```python
from build123d import *

# Parameters (mm, degrees)
SKETCH1_W                 = 82.55
SKETCH1_H                 = 12.7
BOSS_EXTRUDE1_DEPTH       = 3.175
SKETCH3_W                 = 12.7
SKETCH3_H                 = 12.7
BOSS_EXTRUDE2_DEPTH       = 38.1
SKETCH4_W                 = 12.7
SKETCH4_H                 = 12.7
BOSS_EXTRUDE3_DEPTH       = 38.1
SKETCH5_W                 = 6.858
SKETCH5_H                 = 6.858
CUT_EXTRUDE1_DEPTH        = 38.1
SKETCH6_W                 = 6.858
SKETCH6_H                 = 6.858
CUT_EXTRUDE2_DEPTH        = 38.1
SKETCH9_R                 = 2.54
CUT_EXTRUDE3_DEPTH        = 38.1
F_8_32_TAPPED_HOLE2_D     = 3.4544
F_8_32_TAPPED_HOLE2_DEPTH = 2.921


with BuildPart() as part:
    # Sketch1 → Boss-Extrude1 (new body)
    with BuildSketch(Plane(origin=(0, 0, 0), x_dir=(1, 0, 0), z_dir=(0, 1, 0))):
        Rectangle(SKETCH1_W, SKETCH1_H)
    extrude(amount=BOSS_EXTRUDE1_DEPTH)

    # Sketch3 → Boss-Extrude2 (add)
    with BuildSketch(Plane(origin=(0, 3.175, 0), x_dir=(1, 0, 0), z_dir=(0, 1, 0))):
        with Locations((-34.925, 0)):
            Rectangle(SKETCH3_W, SKETCH3_H)
    extrude(amount=BOSS_EXTRUDE2_DEPTH)

    # Sketch4 → Boss-Extrude3 (add)
    with BuildSketch(Plane(origin=(0, 3.175, 0), x_dir=(1, 0, 0), z_dir=(0, 1, 0))):
        with Locations((34.925, 0)):
            Rectangle(SKETCH4_W, SKETCH4_H)
    extrude(amount=BOSS_EXTRUDE3_DEPTH)

    # Sketch5 → Cut-Extrude1 (cut)
    with BuildSketch(Plane(origin=(0, 41.275, 0), x_dir=(1, 0, 0), z_dir=(0, 1, 0))):
        with Locations((-34.925, 0)):
            Rectangle(SKETCH5_W, SKETCH5_H)
    extrude(amount=-CUT_EXTRUDE1_DEPTH, mode=Mode.SUBTRACT)

    # Sketch6 → Cut-Extrude2 (cut)
    with BuildSketch(Plane(origin=(0, 41.275, 0), x_dir=(1, 0, 0), z_dir=(0, 1, 0))):
        with Locations((34.925, 0)):
            Rectangle(SKETCH6_W, SKETCH6_H)
    extrude(amount=-CUT_EXTRUDE2_DEPTH, mode=Mode.SUBTRACT)

    # Sketch9 → Cut-Extrude3 (cut)
    with BuildSketch(Plane(origin=(0, 3.175, 0), x_dir=(1, 0, 0), z_dir=(0, 1, 0))):
        with Locations(Location((-16.51, 0, 0), (0, 0, 270))):
            Circle(SKETCH9_R)
        with Locations(Location((16.51, 0, 0), (0, 0, 270))):
            Circle(SKETCH9_R)
    extrude(amount=-CUT_EXTRUDE3_DEPTH, mode=Mode.SUBTRACT)

    # #8-32 Tapped Hole2
    with Locations(Plane(origin=(-34.925, 36.83, 6.35), x_dir=(1, 0, 0), z_dir=(0, 0, 1))):
        with Locations((0, 0), (69.85, 0)):
            Hole(F_8_32_TAPPED_HOLE2_D / 2, depth=F_8_32_TAPPED_HOLE2_DEPTH)


solid = part.part
```
Here's how the part is built. I have some questions about the finished solid (model axes, mm). A direction names the side the tool comes from. Coordinates: 2 decimals unless noted, no trailing zeros. Loops run counter-clockwise (first coordinate to the right, second up) from the corner with the lowest first, then second, coordinate; pieces in that order, holes last. Notation, with made-up numbers: (16, 48.5) -> (40, 48.5) arc R31 ccw to (40, 76.5) -> close; hole circle Ø4 at (55.5, 78.25). An arc over 180 degrees is marked (long way). Return JSON: item names as keys, results as strings.
1) If we section it at A-A, the plane y = 6: Write out the boundary of the cut face in (x, z) (3 decimals).
Results below:
{"outline": "(-41.275, -6.35) -> (-28.575, -6.35) -> (-28.575, 6.35) -> (-41.275, 6.35) -> close; (28.575, -6.35) -> (41.275, -6.35) -> (41.275, 6.35) -> (28.575, 6.35) -> close; hole (-38.354, -3.429) -> (-31.496, -3.429) -> (-31.496, 3.429) -> (-38.354, 3.429) -> close; hole (31.496, -3.429) -> (38.354, -3.429) -> (38.354, 3.429) -> (31.496, 3.429) -> close"}
2) If we section it at B-B, the plane z = 0: Write out the boundary of the cut face in (x, y) (3 decimals).
Results below:
{"outline": "(-41.275, 0) -> (-19.05, 0) -> (-19.05, 3.175) -> (-28.575, 3.175) -> (-28.575, 41.275) -> (-31.496, 41.275) -> (-31.496, 3.175) -> (-38.354, 3.175) -> (-38.354, 41.275) -> (-41.275, 41.275) -> close; (-13.97, 0) -> (13.97, 0) -> (13.97, 3.175) -> (-13.97, 3.175) -> close; (19.05, 0) -> (41.275, 0) -> (41.275, 41.275) -> (38.354, 41.275) -> (38.354, 3.175) -> (31.496, 3.175) -> (31.496, 41.275) -> (28.575, 41.275) -> (28.575, 3.175) -> (19.05, 3.175) -> close"}
3) Will this pin go through, and if not, where does the flat tip stop? pin 1 (2 mm diameter, centred on x = 36.5, z = -1, fed in from +Y) (3 decimals).
Results below:
{"pin 1": "y = 3.175"}
4) Thinking about a two-plate mould opening in X: for faces 1 (the face through (-41.275, 20, 0)), 2 (the face through (-28.575, 22, 0)), 3 (the face through (-1, 0, 0)), which applies, +X half, -X half, draft (parallel to the pull), parting line (faces both ways), or undercut?
Results below:
{"face 1": "-X half", "face 2": "undercut", "face 3": "draft"}
5) If we section it at C-C, the plane x = -16.51: Write out the boundary of the cut face in (y, z) (3 decimals).
Results below:
{"outline": "(0, -6.35) -> (3.175, -6.35) -> (3.175, -2.54) -> (0, -2.54) -> close; (0, 2.54) -> (3.175, 2.54) -> (3.175, 6.35) -> (0, 6.35) -> close"}
6) For faces 4 (the face through (-34.551, 35.144, 4.869)), 5 (the face through (28.575, 22, 0)), 6 (the face through (-31.496, 22, 0)), which set-ups out of +Z, -Z, +X, -X, +Y, -Y let a thin tool reach every point of the face, with its end or its side?
Results below:
{"face 4": "+Z", "face 5": "+Z, -Z, +Y", "face 6": "+Y"}
7) If we section it at D-D, the plane y = 36.83: Write out the boundary of the cut face in (x, z) (3 decimals).
Results below:
{"outline": "(-41.275, -6.35) -> (-28.575, -6.35) -> (-28.575, 6.35) -> (-33.198, 6.35) -> (-33.198, 3.429) -> (-31.496, 3.429) -> (-31.496, -3.429) -> (-38.354, -3.429) -> (-38.354, 3.429) -> (-36.652, 3.429) -> (-36.652, 6.35) -> (-41.275, 6.35) -> close; (28.575, -6.35) -> (41.275, -6.35) -> (41.275, 6.35) -> (36.652, 6.35) -> (36.652, 3.429) -> (38.354, 3.429) -> (38.354, -3.429) -> (31.496, -3.429) -> (31.496, 3.429) -> (33.198, 3.429) -> (33.198, 6.35) -> (28.575, 6.35) -> close"}
8) I need wall thicknesses on line 1 (X direction, y = 2.3, z = 0) (3 decimals); line 2 (X direction, y = 22, z = -3) (3 decimals); line 3 (X direction, y = 14.5, z = 4) (3 decimals). Which ranges of each line are inside material? Lowest first, please. Write a range as from..to.
Results below:
{"line 1": "-41.275..-19.05, -13.97..13.97, 19.05..41.275", "line 2": "-41.275..-38.354, -31.496..-28.575, 28.575..31.496, 38.354..41.275", "line 3": "-41.275..-28.575, 28.575..41.275"}
